Design review of the part built by this model. Coordinates are the model's own, in mm. Face numbers are marked on the shaded views. A direction names the side the tool comes from. Give positions to 0.01 mm unless a question says otherwise; leave off trailing zeros. Write each loop counter-clockwise with the first axis right and the second up, starting at its lowest first coordinate (ties: lowest second). Pieces come first, ordered by that corner, then holes. Notation, with made-up numbers: (84.5, -10) - (138.5, -10) arc R11 ccw to (138.5, -5) - close; hole circle Ø1 at (-23.5, 73). An arc over 180 degrees is marked (long way). Use a Markdown table: item, result. Add a question column.
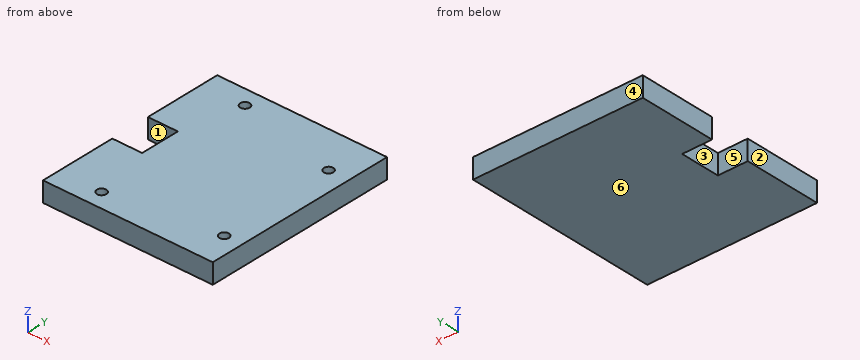
```python
from build123d import *

# Parameters (mm, degrees)
F0_W     = 216
F0_H     = 25.4
F1_DEPTH = 248
F2_R     = 6
F3_DEPTH = 12.7
F4_W     = 38
F4_H     = 50.8
F5_DEPTH = 25.4


with BuildPart() as f1:
    # F0 (on Front) → F1 (new body)
    with BuildSketch(Plane.XZ):
        with Locations((-108, 12.7)):
            Rectangle(F0_W, F0_H)
    extrude(amount=-F1_DEPTH)

    # F2 (on face) → F3 (cut)
    with BuildSketch(Plane.XY.offset(25.4)):
        with Locations((-161, 226)):
            Circle(F2_R)
        with Locations((-161, 22)):
            Circle(F2_R)
        with Locations((-26, 194)):
            Circle(F2_R)
        with Locations((-23, 42)):
            Circle(F2_R)
    extrude(amount=-F3_DEPTH, mode=Mode.SUBTRACT)

    # F4 (on face) → F5 (cut, through all)
    with BuildSketch(Plane.XY.offset(25.4)):
        with Locations((-197, 124)):
            Rectangle(F4_W, F4_H)
    extrude(amount=-F5_DEPTH, mode=Mode.SUBTRACT)


solid = f1.part
```
(1) Add section B-B (z = 18.5). State the section outline as (x, y) points.
(2) Add section C-C (y = 42). State the section outline as (x, z) points.
(3) Add section A-A (x = -182). State the section outline as (y, z) points, and give its area (3 significant figures).
(4) Add section D-D (z = 6.5). State the section outline as (x, y) points, and give its area (3 significant figures).
(5) For line 1 along Y through (x, z) = (-161, 17.75); line 2 along Y through (x, z) = (-183, 20.75); line 3 along Y through (x, z) = (-162, 21.25), list the stretches that pass through material, from the lowest coordinate up.
(6) Tool access review of the marked faces 5 and 6: name each direction out of +Z, -Z, +X, -X, +Y, -Y from which nothing blocks a thin tool from reaching the whole face with its end or side.
(7) Mouldability with a two-part tool opening along Y and no side actions: class the marked faces 1, 2, 3 and 4 as +Y half, -Y half, draft (parallel to the pull), parting line (faces both ways), or undercut.
Answers follow:
| question | item | result |
|---|---|---|
| 1 | outline | (-216, 0) - (0, 0) - (0, 248) - (-216, 248) - (-216, 149.4) - (-178, 149.4) - (-178, 98.6) - (-216, 98.6) - close; hole circle Ø12 at (-161, 22); hole circle Ø12 at (-161, 226); hole circle Ø12 at (-26, 194); hole circle Ø12 at (-23, 42) |
| 2 | outline | (-216, 0) - (0, 0) - (0, 25.4) - (-17, 25.4) - (-17, 12.7) - (-29, 12.7) - (-29, 25.4) - (-216, 25.4) - close |
| 3 | outline | (0, 0) - (98.6, 0) - (98.6, 25.4) - (0, 25.4) - close; (149.4, 0) - (248, 0) - (248, 25.4) - (149.4, 25.4) - close |
| 3 | area | 5,010 mm^2 |
| 4 | outline | (-216, 0) - (0, 0) - (0, 248) - (-216, 248) - (-216, 149.4) - (-178, 149.4) - (-178, 98.6) - (-216, 98.6) - close |
| 4 | area | 51,600 mm^2 |
| 5 | line 1 | 0 to 16, 28 to 220, 232 to 248 |
| 5 | line 2 | 0 to 98.6, 149.4 to 248 |
| 5 | line 3 | 0 to 16.08, 27.92 to 220.08, 231.92 to 248 |
| 6 | face 5 | +Z, -Z, -X |
| 6 | face 6 | -Z, +X, -X, +Y, -Y |
| 7 | face 1 | undercut |
| 7 | face 2 | draft |
| 7 | face 3 | undercut |
| 7 | face 4 | +Y half |
